from build123d import *

# Parameters (mm, degrees)
F0_W     = 127
F0_H     = 190.5
F0_W_2   = 121.92
F0_H_2   = 185.42
F1_DEPTH = 25.4
F2_W     = 121.92
F2_H     = 3.175
F3_DEPTH = 185.42
F4_W     = 121.92
F4_H     = 185.42
F4_W_2   = 116.84
F4_H_2   = 180.34
F5_DEPTH = 10.16
F6_R     = 1.5875
F7_DEPTH = 25.4
F8_R     = 2.54


with BuildPart() as f1:
    # F0 (on Top) → F1 (new body)
    with BuildSketch(Plane.XY):
        Rectangle(F0_W, F0_H)
        Rectangle(F0_W_2, F0_H_2, mode=Mode.SUBTRACT)
    extrude(amount=F1_DEPTH)

    # F2 (on face) → F3 (join)
    with BuildSketch(Plane.XZ.offset(-92.71)):
        with Locations((0, 1.5875)):
            Rectangle(F2_W, F2_H)
    extrude(amount=F3_DEPTH)

    # F4 (on face) → F5 (join)
    with BuildSketch(Plane.XY.offset(3.175)):
        Rectangle(F4_W, F4_H)
        Rectangle(F4_W_2, F4_H_2, mode=Mode.SUBTRACT)
    extrude(amount=F5_DEPTH)

    # F6 (on face) → F7 (cut)
    with BuildSketch(Plane.XY.offset(3.175)):
        with Locations((-53.9496, 85.6996)):
            Circle(F6_R)
        with Locations((53.9496, 85.6996)):
            Circle(F6_R)
        with Locations((-53.9496, -85.6996)):
            Circle(F6_R)
        with Locations((53.9496, -85.6996)):
            Circle(F6_R)
    extrude(amount=-F7_DEPTH, mode=Mode.SUBTRACT)

    # F8
    f8_edges = [f1.edges().sort_by_distance(p)[0] for p in [
        (-63.5, 95.25, 12.7),
        (-63.5, 0, 0),
        (0, 95.25, 0),
        (63.5, 95.25, 12.7),
        (63.5, 0, 0),
        (0, -95.25, 0),
        (63.5, -95.25, 12.7),
        (-63.5, -95.25, 12.7),
    ]]
    fillet(f8_edges, radius=F8_R)


solid = f1.part
Can you work these out from the model? Positions are in its coordinate system, mm. A direction names the side the tool comes from. Coordinates: 2 decimals unless noted, no trailing zeros. Order: outer loops, then holes, each group sorted by start corner. A loop starts at its lowest first (then second) coordinate and runs counter-clockwise, first axis right, second up. Notation, with made-up numbers: (-12.5, -22.75) - (46.5, -22.75) arc R31 ccw to (46.5, 14.25) - close; hole circle Ø1 at (16, 1.25). An arc over 180 degrees is marked (long way). Answer as a JSON object with one key per item and string values. Group by question number.
Q1. Will these pins go through, and if not, where does the flat tip stop? P1, Ø3.5, axis at x = 53.95, y = 85.7, coming from the +Z side (3 decimals); P2, Ø1.9, axis at x = -53.95, y = 85.7, coming from the -Z side.
Q2. Imagine slicing it at D-D (z = 7.25). Please give me the cut outline in (x, y), and give its area (3 significant figures).
Q3. Imagine slicing it at C-C (x = 40). Please give me the cut outline in (y, z) (3 decimals), and give its area (3 significant figures).
Q4. We'd pull the mould along Y, two halves only. Please class faces 1 (the face through (-1, -95.25, 14)), 2 (the face through (60.96, -1, 19)), 3 (the face through (63.5, -1, 14)): +Y half, -Y half, draft (parallel to the pull), parting line (faces both ways), or undercut.
Q5. On a 3-axis mill with a long thin cutter (end or side, diameter ignored), from which of +Z, -Z, +X, -X, +Y, -Y can I reach the whole of each face in a straight line? I mean faces 4 (the face through (-63.5, -1, 14)), 5 (the face through (-1, -92.71, 19)). Say none if no direction works.
Q6. Imagine slicing it at B-B (y = -79.5). Please give me the cut outline in (x, z) (3 decimals).
Q7. I need wall thicknesses on line 1 (X direction, y = 71, z = 15); line 2 (X direction, y = -14, z = 8.75); line 3 (Y direction, x = 36.5, z = 9.5). Which ranges of each line are inside material? Lowest first, please. Write a range as from..to.
Q8. Imagine slicing it at A-A (z = 21). Please give me the cut outline in (x, y).
Determined:
{
 "1": {"P1": "stops at z = 3.175", "P2": "passes through"},
 "2": {"outline": "(-63.5, -92.71) arc R2.54 ccw to (-60.96, -95.25) - (60.96, -95.25) arc R2.54 ccw to (63.5, -92.71) - (63.5, 92.71) arc R2.54 ccw to (60.96, 95.25) - (-60.96, 95.25) arc R2.54 ccw to (-63.5, 92.71) - close; hole (-58.42, -90.17) - (58.42, -90.17) - (58.42, 90.17) - (-58.42, 90.17) - close", "area": "3,120 mm2"},
 "3": {"outline": "(-95.25, 2.54) arc R2.54 ccw to (-92.71, 0) - (92.71, 0) arc R2.54 ccw to (95.25, 2.54) - (95.25, 25.4) - (92.71, 25.4) - (92.71, 13.335) - (90.17, 13.335) - (90.17, 3.175) - (-90.17, 3.175) - (-90.17, 13.335) - (-92.71, 13.335) - (-92.71, 25.4) - (-95.25, 25.4) - close", "area": "767 mm2"},
 "4": {"face 1": "-Y half", "face 2": "undercut", "face 3": "draft"},
 "5": {"face 4": "+Z, -Z, -X, +Y, -Y", "face 5": "+Z"},
 "6": {"outline": "(-63.5, 2.54) arc R2.54 ccw to (-60.96, 0) - (60.96, 0) arc R2.54 ccw to (63.5, 2.54) - (63.5, 25.4) - (60.96, 25.4) - (60.96, 13.335) - (58.42, 13.335) - (58.42, 3.175) - (-58.42, 3.175) - (-58.42, 13.335) - (-60.96, 13.335) - (-60.96, 25.4) - (-63.5, 25.4) - close"},
 "7": {"line 1": "x = -63.5..-60.96, 60.96..63.5", "line 2": "x = -63.5..-58.42, 58.42..63.5", "line 3": "y = -95.25..-90.17, 90.17..95.25"},
 "8": {"outline": "(-63.5, -92.71) arc R2.54 ccw to (-60.96, -95.25) - (60.96, -95.25) arc R2.54 ccw to (63.5, -92.71) - (63.5, 92.71) arc R2.54 ccw to (60.96, 95.25) - (-60.96, 95.25) arc R2.54 ccw to (-63.5, 92.71) - close; hole (-60.96, -92.71) - (60.96, -92.71) - (60.96, 92.71) - (-60.96, 92.71) - close"}
}
